Part print with two shaded views. Sizes in mm from the minimum x, y, z corner. A direction names the side the tool comes from. Coordinates: 2 decimals unless noted, no trailing zeros. Loops run counter-clockwise (first coordinate to the right, second up) from the corner with the lowest first, then second, coordinate; pieces in that order, holes last. Notation, with made-up numbers: (57.5, 55) -> (65.5, 55) arc R19 cw to (65.5, 77) -> close; hole circle Ø6 at (21.25, -11). An arc over 180 degrees is marked (long way). Write each question's results on one line, items separated by ' | '.
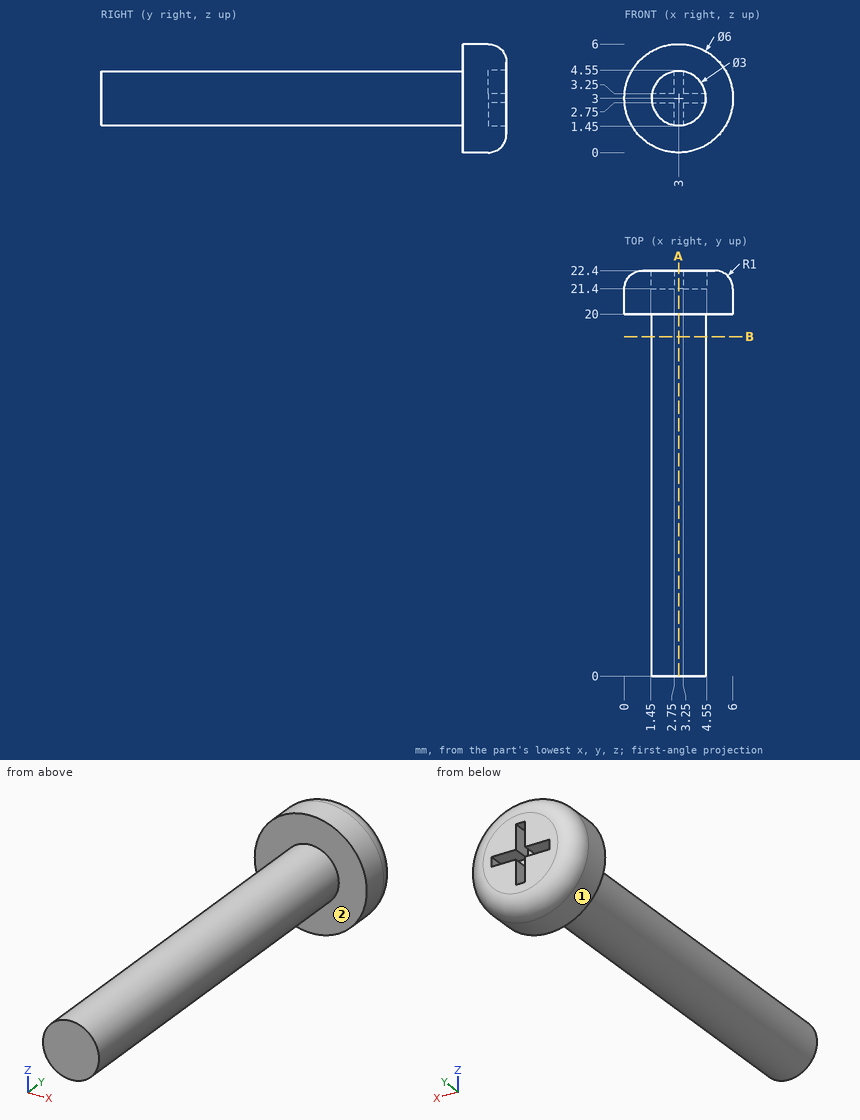
Q1. Cut at A-A on x = 3. Write the cut outline in (y, z), and give its area (3 significant figures).
Results are:
outline: (0, 1.5) -> (20, 1.5) -> (20, 0) -> (21.4, 0) arc R1 ccw to (22.4, 1) -> (22.4, 1.45) -> (21.4, 1.45) -> (21.4, 4.55) -> (22.4, 4.55) -> (22.4, 5) arc R1 ccw to (21.4, 6) -> (20, 6) -> (20, 4.5) -> (0, 4.5) -> close | area: 70.9 mm^2
Q2. Cut at B-B on y = 18.75. Write the cut outline in (x, z).
Results are:
outline: circle Ø3 at (3, 3)
Q3. Drop flat-ended pins along their axis: pin 1 (1.5 mm diameter, centred on x = 2.5, y = 15.5, fed in from -Z); pin 2 (0.5 mm diameter, centred on x = 4, y = 21.5, fed in from +Z); pin 3 (1.1 mm diameter, centred on y = 22, z = 2, fed in from -X). Give the stop position or say it passes through.
Results are:
pin 1: z = 1.5 | pin 2: z = 5.9 | pin 3: x = 0.09
Q4. Which spindle directions (+Z, -Z, +X, -X, +Y, -Y) get a long thin tool onto all of the face, cutting with end or side? Do the marked faces 1 and 2. Say none if no direction does.
Results are:
face 1: +Y, -Y | face 2: -Y
Q5. Wall check: L1, parallel to Y at x = 5, z = 2.75; L2, parallel to X at y = 10.5, z = 2.75; L3, parallel to Y at x = 1.05, z = 4.5. Give the ranges that are in metal, low to high. Write a range as from..to.
Results are:
L1: 20..22.4 | L2: 1.52..4.48 | L3: 20..22.29
